from build123d import *

# Parameters (mm, degrees)
F0_W     = 38.1
F0_H     = 88.9
F1_DEPTH = 444.5
F3_DEPTH = 88.9
F4_R     = 5.08


with BuildPart() as f1:
    # F0 (on Front) → F1 (new body)
    with BuildSketch(Plane.XZ):
        with Locations((2.837234, -1.626216)):
            Rectangle(F0_W, F0_H)
    extrude(amount=F1_DEPTH)

    # F2 (on face) → F3 (cut)
    with BuildSketch(Plane.XY.offset(42.823784)):
        Polygon((21.887234, -406.4), (-16.212766, -444.5), (21.887234, -444.5), align=None)
    extrude(amount=-F3_DEPTH, mode=Mode.SUBTRACT)

    # F4
    f4_edges = [f1.edges().sort_by_distance(p)[0] for p in [
        (21.887234, -203.2, 42.823784),
        (21.887234, -203.2, -46.076216),
        (-16.212766, -222.25, 42.823784),
        (-16.212766, -222.25, -46.076216),
    ]]
    fillet(f4_edges, radius=F4_R)


solid = f1.part
Source: CAD feature listing. Evaluate the final solid. Frame: model axes, mm. Give positions to 0.01 mm unless a question says otherwise; leave off trailing zeros. Order: outer loops, then holes, each group sorted by start corner. A loop starts at its lowest first (then second) coordinate and runs counter-clockwise, first axis right, second up. Notation, with made-up numbers: (-34.5, 73) -> (24.5, 73) arc R28 ccw to (24.5, 104) -> close; hole circle Ø10 at (48.25, -16). An arc over 180 degrees is marked (long way). Use a Markdown table: item, result.
1) Contact query for flat-ended pins moving along their axis: P1, Ø5, axis at x = 7.5, z = -2, coming from the -Y side; P2, Ø1.5, axis at x = 17.5, z = 17, coming from the -Y side. Output: stop coordinate, or through.
Answer list:
| item | result |
|---|---|
| P1 | y = -423.29 |
| P2 | y = -411.54 |
2) Ray query, line 1 along Y through (x, z) = (16, 36); line 2 along Y through (x, z) = (19.5, -25); line 3 along Z through (x, y) = (20.5, -217.5). Return the intervals inside material, ascending. Write a range as [from, to].
Answer list:
| item | result |
|---|---|
| line 1 | [-412.29, 0] |
| line 2 | [-408.79, 0] |
| line 3 | [-44.48, 41.23] |
3) Section query A-A, the plane z = 9. Return the cut outline in (x, y), then the cut area to 3 significant figures.
Answer list:
| item | result |
|---|---|
| outline | (-16.21, -444.5) -> (21.89, -406.4) -> (21.89, 0) -> (-16.21, 0) -> close |
| area | 16,200 mm² |
4) Section query B-B, the plane x = 2.5. Return the cut outline in (y, z), then the cut area to 3 significant figures.
Answer list:
| item | result |
|---|---|
| outline | (-425.79, -46.08) -> (0, -46.08) -> (0, 42.82) -> (-425.79, 42.82) -> close |
| area | 37,900 mm² |
